For this review, take the finished solid that the model builds, in its own axes (mm). A direction names the side the tool comes from. Round coordinates to 2 decimals unless told otherwise and drop trailing zeros. Order: outer loops, then holes, each group sorted by start corner. A loop starts at its lowest first (then second) coordinate and runs counter-clockwise, first axis right, second up.
```python
from build123d import *

# Parameters (mm, degrees)
SKETCH_1_W          = 53
SKETCH_1_H          = 250
SKETCH_1_R          = 2.025
EXTRUDE_1_DEPTH     = 4
SKETCH_2_W          = 13
SKETCH_2_H          = 193.6536947
CUT_EXTRUDE_1_DEPTH = 4
SKETCH_6_R          = 1.525
CUT_EXTRUDE_3_DEPTH = 4
FILLET_1_R          = 3
CUT_EXTRUDE_4_DEPTH = 4
FILLET_2_R          = 3
CUT_EXTRUDE_5_DEPTH = 4
FILLET_3_R          = 3
FILLET_4_R          = 3


with BuildPart() as part:
    # 草图1 → 凸台-拉伸1 (new body)
    with BuildSketch(Plane.XY):
        with Locations((0, 96.82684735)):
            Rectangle(SKETCH_1_W, SKETCH_1_H)
        with Locations((21.5, 23.17315265)):
            Circle(SKETCH_1_R, mode=Mode.SUBTRACT)
        with Locations((21.5, -23.17315265)):
            Circle(SKETCH_1_R, mode=Mode.SUBTRACT)
        with Locations((-21.5, -23.17315265)):
            Circle(SKETCH_1_R, mode=Mode.SUBTRACT)
        with Locations((-21.5, 3.47684735)):
            Circle(SKETCH_1_R, mode=Mode.SUBTRACT)
    extrude(amount=EXTRUDE_1_DEPTH)

    # 草图2 → 切除-拉伸1 (cut)
    with BuildSketch(Plane.XY.offset(4)):
        with Locations((20, 125)):
            Rectangle(SKETCH_2_W, SKETCH_2_H)
    extrude(amount=-CUT_EXTRUDE_1_DEPTH, mode=Mode.SUBTRACT)

    # 草图6 → 切除-拉伸3 (cut)
    with BuildSketch(Plane(origin=(0, 0, 0), x_dir=(-1, 0, 0), z_dir=(0, 0, -1))):
        with Locations((21.5, 216.82684735)):
            Circle(SKETCH_6_R)
        with Locations((1.5, 216.82684735)):
            Circle(SKETCH_6_R)
    extrude(amount=-CUT_EXTRUDE_3_DEPTH, mode=Mode.SUBTRACT)

    # 圆角1
    fillet_1_edges = [part.edges().sort_by_distance(p)[0] for p in [
        (13.5, 221.82684735, 2),
        (26.5, 28.17315265, 2),
        (13.5, 28.17315265, 2),
        (-26.5, 221.82684735, 2),
        (26.5, -28.17315265, 2),
        (-26.5, -28.17315265, 2),
    ]]
    fillet(fillet_1_edges, radius=FILLET_1_R)

    # 草图7 → 切除-拉伸4 (cut)
    with BuildSketch(Plane.XY.offset(4)):
        Polygon((18.5, 18.499246673), (-18.5, 1.551263043), (-18.5, -20.17315265), (18.5, -20.17315265), align=None)
    extrude(amount=-CUT_EXTRUDE_4_DEPTH, mode=Mode.SUBTRACT)

    # 圆角2
    fillet_2_edges = [part.edges().sort_by_distance(p)[0] for p in [
        (18.5, 18.499246673, 2),
        (18.5, -20.17315265, 2),
        (-18.5, -20.17315265, 2),
        (-18.5, 1.551263043, 2),
    ]]
    fillet(fillet_2_edges, radius=FILLET_2_R)

    # 草图8 → 切除-拉伸5 (cut)
    with BuildSketch(Plane(origin=(0, 0, 0), x_dir=(-1, 0, 0), z_dir=(0, 0, -1))):
        Polygon((20.5, 39.291313444), (0.022812462, 18.814125906), (20.5, 9.434476198), align=None)
        Polygon((16.964466094, 42.82684735), (-7.5, 67.291313444), (-7.5, 22.259977323), (-4.826849962, 21.035531294), align=None)
        Polygon((20.5, 46.362381256), (20.5, 95.291313444), (-3.964466094, 70.82684735), align=None)
        Polygon((16.964466094, 98.82684735), (-7.5, 123.291313444), (-7.5, 74.362381256), align=None)
        Polygon((20.5, 102.362381256), (20.5, 151.291313444), (-3.964466094, 126.82684735), align=None)
        Polygon((16.964466094, 154.82684735), (-7.5, 179.291313444), (-7.5, 130.362381256), align=None)
        Polygon((20.5, 158.362381256), (20.5, 207.291313444), (-3.964466094, 182.82684735), align=None)
        Polygon((16.964466094, 210.82684735), (-7.5, 210.82684735), (-7.5, 186.362381256), align=None)
    extrude(amount=-CUT_EXTRUDE_5_DEPTH, mode=Mode.SUBTRACT)

    # 圆角3
    fillet_3_edges = [part.edges().sort_by_distance(p)[0] for p in [
        (4.826849962, 21.035531294, 2),
    ]]
    fillet(fillet_3_edges, radius=FILLET_3_R)

    # 圆角4
    # the kernel refuses this fillet: 3 mm, written as the material it adds along each edge
    with BuildSketch(Plane(origin=(-16.964466094, 98.82684735, 0), x_dir=(0.707106781186547, 0.7071067811865482, 0), z_dir=(0, 0, 1)), Plane(origin=(3.964466094, 126.82684735, 0), x_dir=(-0.7071067811865479, -0.707106781186547, 0), z_dir=(0, 0, 1)), Plane(origin=(7.5, 210.82684735, 0), x_dir=(0, -1, 0), z_dir=(0, 0, 1)), Plane(origin=(-16.964466094, 154.82684735, 0), x_dir=(0.7071067811865442, 0.7071067811865508, 0), z_dir=(0, 0, 1)), Plane(origin=(3.964466094, 182.82684735, 0), x_dir=(-0.7071067811865441, -0.7071067811865508, 0), z_dir=(0, 0, 1))) as fillet_4_piece_1:
        with BuildLine():
            CenterArc((FILLET_4_R, -FILLET_4_R), FILLET_4_R, 90, 90)
            Line((0, -FILLET_4_R), (-FILLET_4_R * 0.02, -FILLET_4_R))
            Line((-FILLET_4_R * 0.02, -FILLET_4_R), (-FILLET_4_R * 0.02, FILLET_4_R * 0.02))
            Line((-FILLET_4_R * 0.02, FILLET_4_R * 0.02), (FILLET_4_R, FILLET_4_R * 0.02))
            Line((FILLET_4_R, FILLET_4_R * 0.02), (FILLET_4_R, 0))
        make_face()
    extrude(amount=4)
    with BuildSketch(Plane(origin=(7.5, 74.362381256, 0), x_dir=(0, 1, 0), z_dir=(0, 0, 1)), Plane(origin=(-20.5, 102.362381256, 0), x_dir=(0.7071067811865476, 0.7071067811865476, 0), z_dir=(0, 0, 1)), Plane(origin=(7.5, 67.291313444, 0), x_dir=(-0.7071067811865478, -0.7071067811865471, 0), z_dir=(0, 0, 1)), Plane(origin=(-16.964466094, 210.82684735, 0), x_dir=(0.7071067811865466, -0.7071067811865486, 0), z_dir=(0, 0, 1)), Plane(origin=(7.5, 130.362381256, 0), x_dir=(0, 1, 0), z_dir=(0, 0, 1)), Plane(origin=(-20.5, 158.362381256, 0), x_dir=(0.707106781186543, 0.707106781186552, 0), z_dir=(0, 0, 1)), Plane(origin=(-20.5, 39.291313444, 0), x_dir=(0, -1, 0), z_dir=(0, 0, 1))) as fillet_4_piece_2:
        with BuildLine():
            CenterArc((FILLET_4_R * 2.41421356237, FILLET_4_R), FILLET_4_R, 135, 135)
            Line((FILLET_4_R * 1.70710678119, FILLET_4_R * 1.70710678119), (FILLET_4_R * 1.69296464556, FILLET_4_R * 1.72124891681))
            Line((FILLET_4_R * 1.69296464556, FILLET_4_R * 1.72124891681), (-FILLET_4_R * 0.0141421356237, FILLET_4_R * 0.0141421356237))
            Line((-FILLET_4_R * 0.0141421356237, FILLET_4_R * 0.0141421356237), (0, -FILLET_4_R * 0.02))
            Line((0, -FILLET_4_R * 0.02), (FILLET_4_R * 2.41421356237, -FILLET_4_R * 0.02))
            Line((FILLET_4_R * 2.41421356237, -FILLET_4_R * 0.02), (FILLET_4_R * 2.41421356237, 0))
        make_face()
    extrude(amount=4)
    with BuildSketch(Plane(origin=(7.5, 123.291313444, 0), x_dir=(0, -1, 0), z_dir=(0, 0, 1)), Plane(origin=(-20.5, 151.291313444, 0), x_dir=(0.707106781186547, -0.707106781186548, 0), z_dir=(0, 0, 1)), Plane(origin=(-20.5, 46.362381256, 0), x_dir=(0, 1, 0), z_dir=(0, 0, 1)), Plane(origin=(-20.5, 95.291313444, 0), x_dir=(0.7071067811865476, -0.7071067811865476, 0), z_dir=(0, 0, 1)), Plane(origin=(7.5, 186.362381256, 0), x_dir=(-0.7071067811865478, 0.7071067811865474, 0), z_dir=(0, 0, 1)), Plane(origin=(7.5, 179.291313444, 0), x_dir=(0, -1, 0), z_dir=(0, 0, 1)), Plane(origin=(-20.5, 207.291313444, 0), x_dir=(0.7071067811865468, -0.7071067811865482, 0), z_dir=(0, 0, 1))) as fillet_4_piece_3:
        with BuildLine():
            CenterArc((FILLET_4_R * 2.41421356237, -FILLET_4_R), FILLET_4_R, 90, 135)
            Line((FILLET_4_R * 1.70710678119, -FILLET_4_R * 1.70710678119), (FILLET_4_R * 1.69296464556, -FILLET_4_R * 1.72124891681))
            Line((FILLET_4_R * 1.69296464556, -FILLET_4_R * 1.72124891681), (-FILLET_4_R * 0.0141421356237, -FILLET_4_R * 0.0141421356237))
            Line((-FILLET_4_R * 0.0141421356237, -FILLET_4_R * 0.0141421356237), (0, FILLET_4_R * 0.02))
            Line((0, FILLET_4_R * 0.02), (FILLET_4_R * 2.41421356237, FILLET_4_R * 0.02))
            Line((FILLET_4_R * 2.41421356237, FILLET_4_R * 0.02), (FILLET_4_R * 2.41421356237, 0))
        make_face()
    extrude(amount=4)
    with BuildSketch(Plane(origin=(-16.964466094, 42.82684735, 0), x_dir=(0.7071067811865487, -0.7071067811865464, 0), z_dir=(0, 0, 1)), Plane(origin=(3.964466094, 70.82684735, 0), x_dir=(-0.707106781186549, 0.707106781186546, 0), z_dir=(0, 0, 1))) as fillet_4_piece_4:
        with BuildLine():
            CenterArc((FILLET_4_R, FILLET_4_R), FILLET_4_R, 180, 90)
            Line((0, FILLET_4_R), (-FILLET_4_R * 0.02, FILLET_4_R))
            Line((-FILLET_4_R * 0.02, FILLET_4_R), (-FILLET_4_R * 0.02, -FILLET_4_R * 0.02))
            Line((-FILLET_4_R * 0.02, -FILLET_4_R * 0.02), (FILLET_4_R, -FILLET_4_R * 0.02))
            Line((FILLET_4_R, -FILLET_4_R * 0.02), (FILLET_4_R, 0))
        make_face()
    extrude(amount=4)
    with BuildSketch(Plane(origin=(7.5, 22.259977323, 0), x_dir=(-0.9091611234166711, -0.4164445361242436, 0), z_dir=(0, 0, 1))) as fillet_4_piece_5:
        with BuildLine():
            CenterArc((2.03672897, -2.757354466), FILLET_4_R, 113.202499131, 42.187182076)
            Line((-0.6907544, -1.508020858), (-0.745304068, -1.483034186))
            Line((-0.745304068, -1.483034186), (-0.054549667, 0.024986672))
            Line((-0.054549667, 0.024986672), (0, 0.06))
            ThreePointArc((0, 0.06), (0.427391485, 0.06), (0.83114405, 0.055147089))
            Line((0.83114405, 0.055147089), (0.85478297, 0))
        make_face()
    extrude(amount=4)
    with BuildSketch(Plane(origin=(-0.022812462, 18.814125906, 0), x_dir=(-0.9091611234134724, -0.4164445361312268, 0), z_dir=(0, 0, 1))) as fillet_4_piece_6:
        with BuildLine():
            CenterArc((FILLET_4_R * 1.43853500921, -FILLET_4_R), FILLET_4_R, 90, 110.389681207)
            Line((FILLET_4_R * 0.501190258162, -FILLET_4_R * 1.34840324007), (FILLET_4_R * 0.482443363141, -FILLET_4_R * 1.35537130487))
            Line((FILLET_4_R * 0.482443363141, -FILLET_4_R * 1.35537130487), (-FILLET_4_R * 0.0287707001841, FILLET_4_R * 0.02))
            Line((-FILLET_4_R * 0.0287707001841, FILLET_4_R * 0.02), (FILLET_4_R * 1.43853500921, FILLET_4_R * 0.02))
            Line((FILLET_4_R * 1.43853500921, FILLET_4_R * 0.02), (FILLET_4_R * 1.43853500921, 0))
        make_face()
    extrude(amount=4)
    with BuildSketch(Plane(origin=(-20.5, 9.434476198, 0), x_dir=(0, 1, 0), z_dir=(0, 0, 1))) as fillet_4_piece_7:
        with BuildLine():
            CenterArc((FILLET_4_R * 1.55796865886, -FILLET_4_R), FILLET_4_R, 90, 114.610318793)
            Line((FILLET_4_R * 0.648807535446, -FILLET_4_R * 1.41644453613), (FILLET_4_R * 0.630624312977, -FILLET_4_R * 1.42477342685))
            Line((FILLET_4_R * 0.630624312977, -FILLET_4_R * 1.42477342685), (-FILLET_4_R * 0.0311593731772, FILLET_4_R * 0.02))
            Line((-FILLET_4_R * 0.0311593731772, FILLET_4_R * 0.02), (FILLET_4_R * 1.55796865886, FILLET_4_R * 0.02))
            Line((FILLET_4_R * 1.55796865886, FILLET_4_R * 0.02), (FILLET_4_R * 1.55796865886, 0))
        make_face()
    extrude(amount=4)


solid = part.part
```
Q1. Clearance check with flat-ended pins moving along their axes: pin 1 (10 mm diameter, centred on x = 1.5, y = 109.5, fed in from -Z); pin 2 (2 mm diameter, centred on y = 135, z = 2.5, fed in from +X). State where each tip first meets the part, or that it passes through.
Q2. Take a section at B-B, the plane z = 3.2. Count the separate pieces of the cut face and the enclosed holes in it, plus the area to 3 significant figures.
Q3. Tool access review of faces 3 (the face through (-7, 221.827, 2)), 4 (the face through (-6.647, 172.215, 1.972)): name each direction out of +Z, -Z, +X, -X, +Y, -Y from which nothing blocks a thin tool from reaching the whole face with its end or side.
Q4. Take a section at A-A, the plane y = 198. State the section outline as (x, z) points, plus the area to 3 significant figures.
Q5. Mouldability with a two-part tool opening along X and no side actions: class faces 1 (the face through (20, 28.173, 2)), 2 (the face through (-15.72, 98.86, 1.97)) as +X half, -X half, draft (parallel to the pull), parting line (faces both ways), or undercut.
Q6. Wall thickness on line 1 (Y direction, x = 21.5, z = 1.6); line 2 (Y direction, x = -21.5, z = 3.1); line 3 (Y direction, x = -18, z = 2.8): over which ranges is each line inside the solid? List them lowest first.
Working result:
1. pin 1: passes through
1. pin 2: stops at x = 13.5
2. separate pieces: 1
2. enclosed holes: 15
2. area: 5,540 mm2
3. face 3: +Z, -Z, +X, -X, +Y
3. face 4: +Z, -Z
4. outline: (-26.5, 0) - (-20.5, 0) - (-20.5, 4) - (-26.5, 4) - close; (-11.21, 0) - (-4.14, 0) - (-4.14, 4) - (-11.21, 4) - close; (7.5, 0) - (13.5, 0) - (13.5, 4) - (7.5, 4) - close
4. area: 76.3 mm2
5. face 1: draft
5. face 2: undercut
6. line 1: y = -28.17 to -25.2, -21.15 to 21.15, 25.2 to 28.17
6. line 2: y = -28.17 to -25.2, -21.15 to 1.45, 5.5 to 215.3, 218.35 to 221.83
6. line 3: y = -28.17 to -18.83, 1.28 to 11.15, 35.01 to 50.65, 91.01 to 106.65, 147.01 to 162.65, 203.01 to 221.83
